Part print with two shaded views. Sizes in mm from the minimum x, y, z corner. Give positions to 0.01 mm unless a question says otherwise; leave off trailing zeros. Order: outer loops, then holes, each group sorted by start corner. A loop starts at its lowest first (then second) coordinate and runs counter-clockwise, first axis right, second up. Notation, with made-up numbers: M 82,28.5 L 123,28.5 A27 ccw 123,55.5 Z; hole C 76.5,-37 d10. An arc over 180 degrees is marked long. Return JSON: item names as keys, results as strings. Group by question number.
1. Wall check: probe 1 along Z at (x, y) = (13.97, 0.95); probe 2 along Z at (x, y) = (66.5, 0.3); probe 3 along X at (y, z) = (1.35, 46.5). Give the ranges that are in metal, low to high. Write a range as [from, to].
2. Slice it at B-B on z = 17.78. List the corners of the cut face in (x, y).
3. Pin check, flat tip, straight feed: pin 1 (0.5 mm diameter, centred on y = 0.5, z = 51, fed in from +X). Stop position of the tip, or through.
4. Slice it at A-A on y = 0.4. List the corners of the cut face in (x, z) (1 decimal).
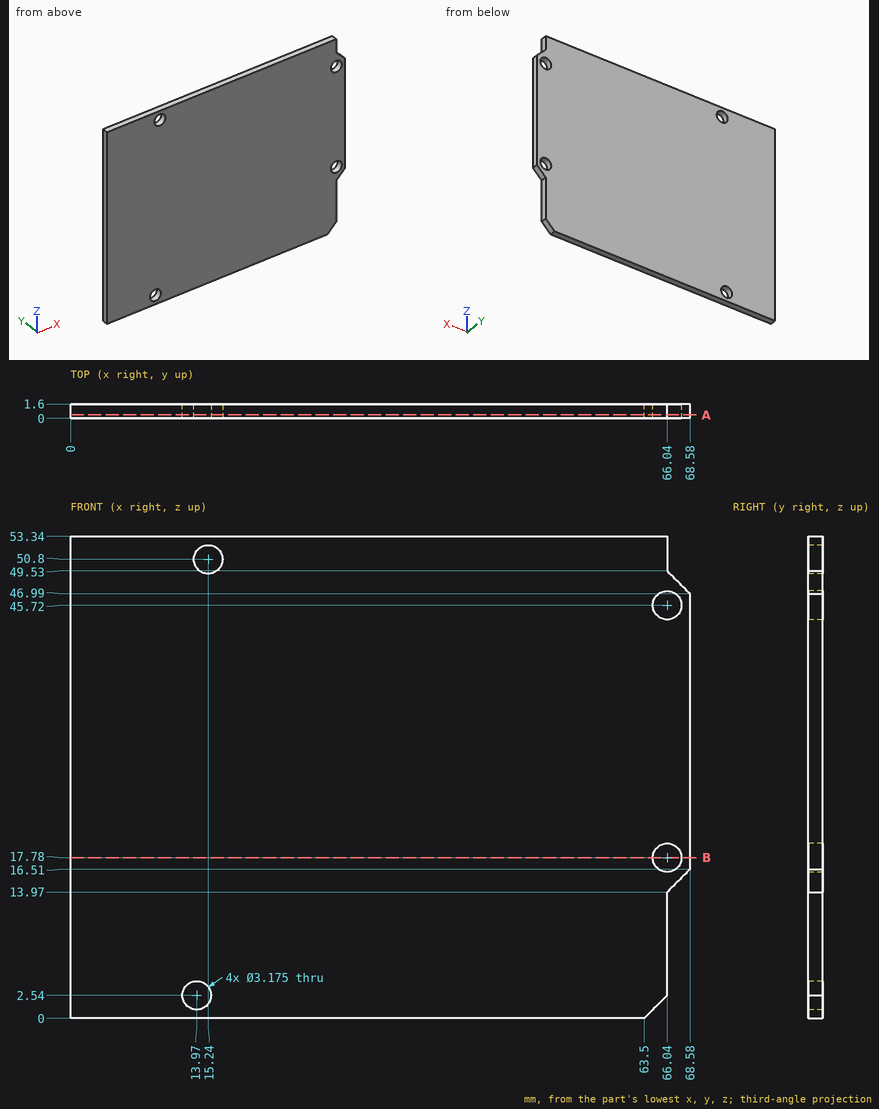
Result:
{
 "1": {"probe 1": "z = [0, 0.95], [4.13, 49.85], [51.75, 53.34]", "probe 2": "z = [14.43, 16.26], [19.3, 44.2], [47.24, 49.07]", "probe 3": "x = [0, 64.66], [67.42, 68.58]"},
 "2": {"outline": "M 0,0 L 64.45,0 L 64.45,1.6 L 0,1.6 Z; M 67.63,0 L 68.58,0 L 68.58,1.6 L 67.63,1.6 Z"},
 "3": {"pin 1": "stops at x = 66.04"},
 "4": {"outline": "M 0,0 L 63.5,0 L 66,2.5 L 66,14 L 68.6,16.5 L 68.6,47 L 66,49.5 L 66,53.3 L 0,53.3 Z; hole C 14,2.5 d3.2; hole C 15.2,50.8 d3.2; hole C 66,17.8 d3.2; hole C 66,45.7 d3.2"}
}
